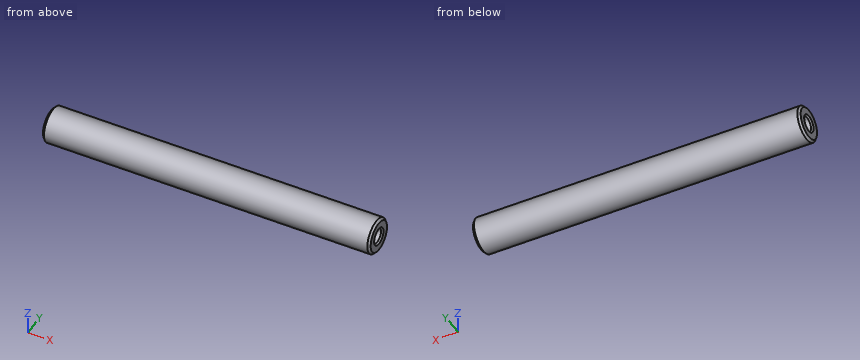
Autodesk Inventor part; units mm, degrees
ref_plane "YZ Plane" through (0, 0, 0) normal (1, 0, 0) x (0, 1, 0)
ref_plane "XZ Plane" through (0, 0, 0) normal (0, 1, 0) x (-1, 0, 0)
ref_plane "XY Plane" through (0, 0, 0) normal (0, 0, 1) x (1, 0, 0)
sketch "Sketch_1" plane through (0, 0, 0) normal (0, 0, 1) x (1, 0, 0)
  line L0 (75.7, 0) -> (0, 0)
  line L1 (0, 0) -> (0, 3.5)
  line L2 (0, 3.5) -> (0.5, 4)
  line L3 (0.5, 4) -> (75.2, 4)
  line L4 (75.2, 4) -> (75.7, 3.5)
  line L5 (75.7, 3.5) -> (75.7, 0)
  line L6 (75.7, 0) -> (0, 0)
revolve "Revolution1" add sketch "Sketch_1" angle 360 about axis through (75.7, 0, 0) along (1, 0, 0)
sketch "Sketch2" plane through (0, 0, 0) normal (-1, 0, 0) x (0, 0, 1)
  point P0 (0, 0)
hole "Hole1" at (0, 0, 0) direction (1, 0, 0) diameter 3.242 depth 13.0641 tip angle 120 countersink diameter 4 countersink angle 90
sketch "Sketch3" plane through (75.7, 0, 0) normal (1, 0, 0) x (0, 0, -1)
  point P0 (0, 0)
hole "Hole2" at (75.7, 0, 0) direction (-1, 0, 0) diameter 3.242 depth 13.0641 tip angle 120 countersink diameter 4 countersink angle 90
properties part number "SFHRW8-75_7-M4-N4_s" material "鋼、炭素鋼"
Can you work these out from the model? Positions are in its coordinate system, mm. Give positions to 0.01 mm unless a question says otherwise; leave off trailing zeros. Order: outer loops, then holes, each group sorted by start corner. A loop starts at its lowest first (then second) coordinate and runs counter-clockwise, first axis right, second up. Notation, with made-up numbers: (67.25, 84) - (119.25, 84) arc R20 ccw to (119.25, 102) - close; hole circle Ø4 at (-23.75, 33.25). An arc over 180 degrees is marked (long way). Use a Markdown table: item, result. Add a question column.
Q1. Please list where these lines run through material, in increasing order: line 1 along Z through (x, y) = (7.5, 0); line 2 along Y through (x, z) = (10, 0.75); line 3 along Z through (x, y) = (65, -0.5).
Q2. If we section it at A-A on x = 64: Write out the boundary of the cut face in (y, z).
Q3. I'm going to push flat-ended pins straight in: pin 1 (2 mm diameter, centred on x = 8, z = -3, fed in from -Y); pin 2 (1 mm diameter, centred on x = 64, z = -1.5, fed in from -Y); pin 3 (3 mm diameter, centred on y = 0, z = 0, fed in from -X). Where does each tip first touch, or does it pass through?
Answers follow:
| question | item | result |
|---|---|---|
| 1 | line 1 | z = -4 to -1.62, 1.62 to 4 |
| 1 | line 2 | y = -3.93 to -1.44, 1.44 to 3.93 |
| 1 | line 3 | z = -3.97 to -1.54, 1.54 to 3.97 |
| 2 | outline | circle Ø8 at (0, 0); hole circle Ø3.24 at (0, 0) |
| 3 | pin 1 | stops at y = -3.46 |
| 3 | pin 2 | stops at y = -3.87 |
| 3 | pin 3 | stops at x = 13.13 |
